Verification items for the finished model (mm, model axes). Face numbers are marked on the shaded views. Coordinates: 2 decimals unless noted, no trailing zeros. Order: outer loops, then holes, each group sorted by start corner. A loop starts at its lowest first (then second) coordinate and runs counter-clockwise, first axis right, second up. Notation, with made-up numbers: M -34.75,30 L 21.25,30 A13 cw 21.25,45 Z; hole C 33,45.5 d3. An arc over 180 degrees is marked long. Answer as a JSON object with one key per item and string values. Group by question number.
(1) Mould release check, pull along X, two halves, no side actions. Record for the marked faces 1, 2, 3 and 4: released by +X, released by -X, zero draft, split by the parting line, or undercut.
(2) Cross-section at C-C (x = -20.5). Enter the section's corners in (y, z), plus the area to 3 significant figures.
(3) Cross-section at D-D (x = -2.5). Enter the section's corners in (y, z), plus the area to 3 significant figures.
(4) Gauge pin test, flat ends, axial feed: pin 1 Ø6 at (y, z) = (-5.5, -5) entering from -X; pin 2 Ø2 at (x, y) = (-3, 4.5) entering from -Z; pin 3 Ø5 at (x, y) = (2, 12) entering from +Z. Record the tip position at first contact, or that the pin passes through.
(5) Material ranges on line 1 (Y direction, x = 0, z = -18.85); line 2 (Z direction, x = 11, y = 23.5); line 3 (X direction, y = -9, z = -2), recorded low to high.
(6) Cross-section at A-A (y = 0). Enter the section's corners in (x, z).
(7) Cross-section at B-B (z = -5). Enter the section's corners in (x, y), plus the area to 3 significant figures.
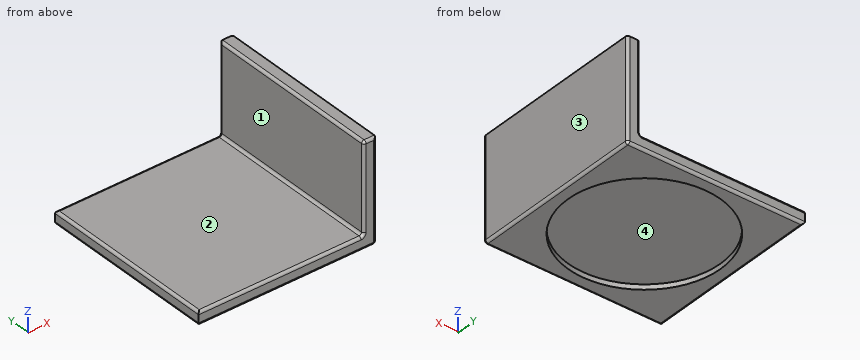
from build123d import *

# Parameters (mm, degrees)
PAD_DEPTH      = 35
PAD_DEPTH_BACK = 35
FILLET_R       = 1
SKETCH001_R    = 30
POCKET_DEPTH   = 2


with BuildPart() as part:
    # Sketch → Pad (new body, two sides)
    with BuildSketch(Plane.XZ) as pad_sk:
        Polygon((-35, -20), (35, -20), (35, 20), (30, 20), (30, -15), (-35, -15), align=None)
    extrude(amount=PAD_DEPTH)
    extrude(pad_sk.sketch, amount=-PAD_DEPTH_BACK)

    # Fillet
    fillet_edges = [part.edges().sort_by_distance(p)[0] for p in [
        (35, 0, -20),
        (-2.5, 35, -15),
        (35, 35, 0),
        (0, 35, -20),
        (-35, 0, -20),
        (-35, 0, -15),
        (-2.5, -35, -15),
        (0, -35, -20),
        (30, -35, 2.5),
        (30, 0, -15),
        (30, 35, 2.5),
        (30, 0, 20),
        (32.5, -35, 20),
        (35, -35, 0),
    ]]
    fillet(fillet_edges, radius=FILLET_R)

    # Sketch001 → Pocket (cut)
    with BuildSketch(Plane.XY.offset(-20)):
        Circle(SKETCH001_R)
    extrude(amount=POCKET_DEPTH, mode=Mode.SUBTRACT)


solid = part.part
Taken from the geometry:
{
 "1": {"face 1": "released by -X", "face 2": "zero draft", "face 3": "released by +X", "face 4": "undercut"},
 "2": {"outline": "M -35,-19 A1 ccw -34,-20 L -21.9,-20 L -21.9,-18 L 21.9,-18 L 21.9,-20 L 34,-20 A1 ccw 35,-19 L 35,-16 A1 ccw 34,-15 L -34,-15 A1 ccw -35,-16 Z", "area": "262 mm²"},
 "3": {"outline": "M -35,-19 A1 ccw -34,-20 L -29.9,-20 L -29.9,-18 L 29.9,-18 L 29.9,-20 L 34,-20 A1 ccw 35,-19 L 35,-16 A1 ccw 34,-15 L -34,-15 A1 ccw -35,-16 Z", "area": "230 mm²"},
 "4": {"pin 1": "stops at x = 30", "pin 2": "stops at z = -18", "pin 3": "stops at z = -15"},
 "5": {"line 1": "y = -35 to -30, 30 to 35", "line 2": "z = -18 to -15", "line 3": "x = 30 to 35"},
 "6": {"outline": "M -35,-19 A1 ccw -34,-20 L -30,-20 L -30,-18 L 30,-18 L 30,-20 L 34,-20 A1 ccw 35,-19 L 35,20 L 31,20 A1 ccw 30,19 L 30,-14 A1 cw 29,-15 L -34,-15 A1 ccw -35,-16 Z"},
 "7": {"outline": "M 30,-34 A1 ccw 31,-35 L 34,-35 A1 ccw 35,-34 L 35,34 A1 ccw 34,35 L 31,35 A1 ccw 30,34 Z", "area": "349 mm²"}
}
